Source: CAD feature listing. Evaluate the final solid. Frame: model axes, mm. Give positions to 0.01 mm unless a question says otherwise; leave off trailing zeros. Write each loop counter-clockwise with the first axis right and the second up, starting at its lowest first coordinate (ties: lowest second). Pieces come first, ordered by that corner, then holes.
```python
from build123d import *

# Parameters (mm, degrees)
GENERAL_SHAPE_DEPTH        = 1.6
M2_CLEARANCE_HOLE1_D       = 2.6
MIRROR2_COPY_1_D           = 2.6
SKETCH5_R                  = 0.8
CONNECTOR_HOLES_DEPTH      = 89.897525275
STAR_TRACKER_CUTOUTS_DEPTH = 89.897525275


with BuildPart() as part:
    # Sketch1 → General Shape (new body)
    with BuildSketch(Plane.XY):
        with BuildLine():
            Line((-38.5, 78.6), (38.5, 78.6))
            ThreePointArc((38.5, 78.6), (40.621320344, 77.721320344), (41.5, 75.6))
            Line((41.5, 75.6), (41.5, -75.6))
            ThreePointArc((41.5, -75.6), (40.621320344, -77.721320344), (38.5, -78.6))
            Line((38.5, -78.6), (-38.5, -78.6))
            ThreePointArc((-38.5, -78.6), (-40.621320344, -77.721320344), (-41.5, -75.6))
            Line((-41.5, -75.6), (-41.5, 75.6))
            ThreePointArc((-41.5, 75.6), (-40.621320344, 77.721320344), (-38.5, 78.6))
        make_face()
    extrude(amount=GENERAL_SHAPE_DEPTH)

    # M2 Clearance Hole1 (through all)
    with Locations(Plane(origin=(-39.5, 73.6, 0), x_dir=(-1, 0, 0), z_dir=(0, 0, -1))):
        with Locations((0, 0), (0, -28.4), (0, -56.8)):
            m2_clearance_hole1 = Hole(M2_CLEARANCE_HOLE1_D / 2)

    # Mirror1: M2 Clearance Hole1 across plane
    add(m2_clearance_hole1.mirror(Plane(origin=(0, 0, 0), x_dir=(0, 0, 1), z_dir=(1, 0, 0))), mode=Mode.SUBTRACT)

    # Mirror2: M2 Clearance Hole1 across plane
    add(m2_clearance_hole1.mirror(Plane.ZX), mode=Mode.SUBTRACT)

    # Mirror2 copy 1 (through all)
    with Locations(Plane(origin=(39.5, -73.6, 0), x_dir=(1, 0, 0), z_dir=(0, 0, -1))):
        with Locations((0, 0), (0, -28.4), (0, -56.8)):
            Hole(MIRROR2_COPY_1_D / 2)

    # Sketch5 → Connector holes (cut, through all)
    with BuildSketch(Plane(origin=(0, 0, 0), x_dir=(-1, 0, 0), z_dir=(0, 0, -1))):
        with Locations((-5.38, 70.6)):
            Circle(SKETCH5_R)
        with Locations((5.38, 70.6)):
            Circle(SKETCH5_R)
    extrude(amount=-CONNECTOR_HOLES_DEPTH, mode=Mode.SUBTRACT)

    # Sketch6 → Star Tracker Cutouts (cut, through all)
    with BuildSketch(Plane(origin=(0, 0, 0), x_dir=(-1, 0, 0), z_dir=(0, 0, -1))):
        with BuildLine():
            Line((-35.5, 36.6), (-29.5, 36.6))
            ThreePointArc((-29.5, 36.6), (-28.085786438, 36.014213562), (-27.5, 34.6))
            Line((-27.5, 34.6), (-27.5, 23))
            ThreePointArc((-27.5, 23), (-28.085786438, 21.585786438), (-29.5, 21))
            Line((-29.5, 21), (-35.5, 21))
            ThreePointArc((-35.5, 21), (-36.914213562, 21.585786438), (-37.5, 23))
            Line((-37.5, 23), (-37.5, 34.6))
            ThreePointArc((-37.5, 34.6), (-36.914213562, 36.014213562), (-35.5, 36.6))
        make_face()
        with BuildLine():
            Line((29.5, 36.6), (35.5, 36.6))
            ThreePointArc((35.5, 36.6), (36.914213562, 36.014213562), (37.5, 34.6))
            Line((37.5, 34.6), (37.5, 23))
            ThreePointArc((37.5, 23), (36.914213562, 21.585786438), (35.5, 21))
            Line((35.5, 21), (29.5, 21))
            ThreePointArc((29.5, 21), (28.085786438, 21.585786438), (27.5, 23))
            Line((27.5, 23), (27.5, 34.6))
            ThreePointArc((27.5, 34.6), (28.085786438, 36.014213562), (29.5, 36.6))
        make_face()
        with BuildLine():
            Line((-35.5, -21), (-29.5, -21))
            ThreePointArc((-29.5, -21), (-28.085786438, -21.585786438), (-27.5, -23))
            Line((-27.5, -23), (-27.5, -34.6))
            ThreePointArc((-27.5, -34.6), (-28.085786438, -36.014213562), (-29.5, -36.6))
            Line((-29.5, -36.6), (-35.5, -36.6))
            ThreePointArc((-35.5, -36.6), (-36.914213562, -36.014213562), (-37.5, -34.6))
            Line((-37.5, -34.6), (-37.5, -23))
            ThreePointArc((-37.5, -23), (-36.914213562, -21.585786438), (-35.5, -21))
        make_face()
        with BuildLine():
            Line((29.5, -21), (35.5, -21))
            ThreePointArc((35.5, -21), (36.914213562, -21.585786438), (37.5, -23))
            Line((37.5, -23), (37.5, -34.6))
            ThreePointArc((37.5, -34.6), (36.914213562, -36.014213562), (35.5, -36.6))
            Line((35.5, -36.6), (29.5, -36.6))
            ThreePointArc((29.5, -36.6), (28.085786438, -36.014213562), (27.5, -34.6))
            Line((27.5, -34.6), (27.5, -23))
            ThreePointArc((27.5, -23), (28.085786438, -21.585786438), (29.5, -21))
        make_face()
    extrude(amount=-STAR_TRACKER_CUTOUTS_DEPTH, mode=Mode.SUBTRACT)


solid = part.part
```
1. Cut plane A-A, the plane y = -25.5. Return the cut outline in (x, z), then the cut area to 3 significant figures.
2. Contact query for a flat-ended pin moving along its axis: P1, Ø2, axis at x = 39.5, y = -73.6, coming from the -Z side. Output: stop coordinate, or through.
3. Line query: L1, parallel to X at y = 16.8, z = 0.7; L2, parallel to Y at x = -32.5, z = 0.9; L3, parallel to X at y = 30.5, z = 0.25. Output: solid intervals per line, ascending.
4. Cut plane B-B, the plane z = 0.95. State how many separate pieces and enclosed holes the cut face has, then the cut area to 3 significant figures.
Response values:
1. outline: (-41.5, 0) - (-37.5, 0) - (-37.5, 1.6) - (-41.5, 1.6) - close; (-27.5, 0) - (27.5, 0) - (27.5, 1.6) - (-27.5, 1.6) - close; (37.5, 0) - (41.5, 0) - (41.5, 1.6) - (37.5, 1.6) - close
1. area: 101 mm2
2. P1: passes through
3. L1: x = -41.5 to -40.8, -38.2 to 38.2, 40.8 to 41.5
3. L2: y = -78.6 to -36.6, -21 to 21, 36.6 to 78.6
3. L3: x = -41.5 to -37.5, -27.5 to 27.5, 37.5 to 41.5
4. separate pieces: 1
4. enclosed holes: 18
4. area: 12,400 mm2
